CAD build for the part. Positions are in the model's coordinates, mm. Face numbers are marked on the shaded views. A direction names the side the tool comes from. Coordinates: 2 decimals unless noted, no trailing zeros. Loops run counter-clockwise (first coordinate to the right, second up) from the corner with the lowest first, then second, coordinate; pieces in that order, holes last. Notation, with made-up numbers: (-14.75, -34) -> (-4.75, -34) arc R15 cw to (-4.75, -5) -> close; hole circle Ø11 at (81.5, 71.5). An arc over 180 degrees is marked (long way). Answer as a JSON object with one key per item and string values. Group by question number.
from build123d import *

# Parameters (mm, degrees)
BOSS_EXTRUDE1_DEPTH = 40
SKETCH3_R           = 13.5
BOSS_EXTRUDE2_DEPTH = 35
SKETCH4_R           = 11
CUT_EXTRUDE1_DEPTH  = 35


with BuildPart() as part:
    # Sketch2 → Boss-Extrude1 (new body)
    with BuildSketch(Plane.XY):
        Polygon((0, 0), (40, 28.008301528), (40, 0), align=None)
    extrude(amount=BOSS_EXTRUDE1_DEPTH)

    # Sketch3 → Boss-Extrude2 (add)
    with BuildSketch(Plane(origin=(0, 0, 0), x_dir=(0.819152044, 0.573576436, 0), z_dir=(-0.573576436, 0.819152044, 0))):
        with Locations((24.415, -19.983681398)):
            Circle(SKETCH3_R)
    extrude(amount=BOSS_EXTRUDE2_DEPTH)

    # Sketch4 → Cut-Extrude1 (cut)
    with BuildSketch(Plane(origin=(-20.075175272, 28.67032155, 0), x_dir=(0.819152044, 0.573576436, 0), z_dir=(-0.573576436, 0.819152044, 0))):
        with Locations((24.415, -19.983681398)):
            Circle(SKETCH4_R)
    extrude(amount=-CUT_EXTRUDE1_DEPTH, mode=Mode.SUBTRACT)


solid = part.part
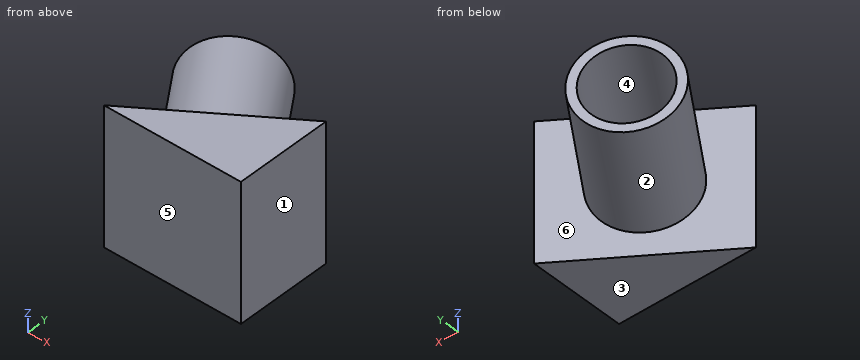
Item 1: Pull direction Z, two halves, no side cores. Call the marked faces 1, 2, 3 and 4: +Z half, -Z half, draft (parallel to the pull), parting line (faces both ways), or undercut.
Item 2: Band-saw the part on C-C, the plane z = 3. List the corners of the cut face in (x, y), and give its area (3 significant figures).
Item 3: Flat gauge pins, fed straight in: P1, Ø1.5, axis at y = 10, z = 18, coming from the -X side; P2, Ø5, axis at y = 43.5, z = 21.5, coming from the -X side; P3, Ø10, axis at x = 3, y = 32.5, coming from the +Z side. Where does each tip first touch, or does it go through?
Item 4: Band-saw the part on D-D, the plane z = 13. List the corners of the cut face in (x, y), and give its area (3 significant figures).
Item 5: Drill centre lines: L1, parallel to X at y = 27.5, z = 25; L2, parallel to Z at x = 5, y = 34.5; L3, parallel to Y at x = 9, z = 28. Where is each one in solid material? Low to high.
Item 6: Band-saw the part on B-B, the plane y = 3.5. List the corners of the cut face in (x, z).
Item 7: 3-axis set-ups, long thin cutter, end or side, ignore diameter. For the marked faces 5 and 6: which of +Z, -Z, +X, -X, +Y, -Y reach the whole face in a straight line?
Item 8: Band-saw the part on A-A, the plane z = 32.5. List the corners of the cut face in (x, y).
Reply:
{
 "1": {"face 1": "draft", "face 2": "parting line", "face 3": "-Z half", "face 4": "undercut"},
 "2": {"outline": "(0, 0) -> (40, 0) -> (40, 28.01) -> close", "area": "560 mm²"},
 "3": {"P1": "x = 5.96", "P2": "x = 10.81", "P3": "z = 33.48"},
 "4": {"outline": "(-9.54, 36.05) -> (10.54, 7.38) -> (0, 0) -> (40, 0) -> (40, 28.01) -> (29.46, 20.63) -> (9.39, 49.3) -> (6.89, 47.55) -> (26.96, 18.88) -> (13.04, 9.13) -> (-7.04, 37.8) -> close", "area": "774 mm²"},
 "5": {"L1": "-4.75 to -1.4, 22.5 to 25.85, 39.27 to 40", "L2": "6.49 to 9, 30.97 to 33.47", "L3": "0 to 6.3, 10.78 to 16.58, 42.85 to 48.65"},
 "6": {"outline": "(5, 0) -> (40, 0) -> (40, 40) -> (5, 40) -> close"},
 "7": {"face 5": "+Z, -Z, +X, -X, -Y", "face 6": "none"},
 "8": {"outline": "(-4.22, 39.77) -> (15.86, 11.1) -> (0, 0) -> (40, 0) -> (40, 28.01) -> (24.14, 16.91) -> (4.07, 45.58) -> close"}
}
